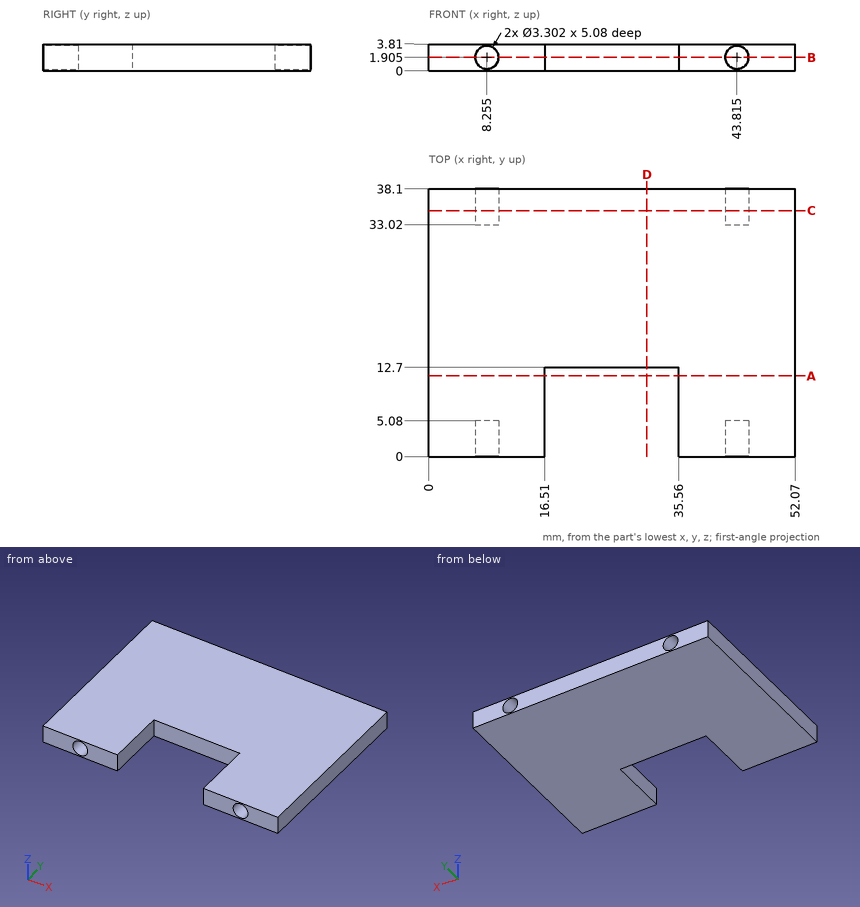
Input: dimensioned drawing with shaded views. Units: mm. Origin: part minimum x, y, z. Coordinates: 2 decimals unless noted, no trailing zeros. Loops run counter-clockwise (first coordinate to the right, second up) from the corner with the lowest first, then second, coordinate; pieces in that order, holes last. Notation, with made-up numbers: M -38,-10.5 L -22,-10.5 A20 cw -22,-6.5 Z; hole C -24,64.25 d2. An arc over 180 degrees is marked long. One line per item, written item: value. Start each with the question number.
1) Cut plane B-B (z = 1.9). Return loops of the section in (x, y), then the cut area to 3 significant figures.
2) Cut plane D-D (x = 31). Return loops of the section in (y, z).
3) Pin query (flat end, axial travel): P1, Ø1.7, axis at x = 44, z = 2.5, coming from the +Y side; P2, Ø2, axis at x = 43.815, z = 1.905, coming from the -Y side; P3, Ø1, axis at x = 19.5, z = 2.5, coming from the -Y side; P4, Ø1.7, axis at x = 44.5, z = 2.5, coming from the -Y side. Return the tip coordinate at first contact, or that it passes through.
4) Cut plane C-C (y = 35). Return loops of the section in (x, z) (3 decimals).
5) Material intervals for L1, parallel to X at y = 2.5, z = 1.95; L2, parallel to X at y = 11, z = 0.35; L3, parallel to Y at x = 31.5, z = 0.9, sorted ascending. Write a range as from..to.
6) Cut plane A-A (y = 11.5). Return loops of the section in (x, z), then the cut area to 3 significant figures.
Evaluation:
1. outline: M 0,0 L 6.6,0 L 6.6,5.08 L 9.91,5.08 L 9.91,0 L 16.51,0 L 16.51,12.7 L 35.56,12.7 L 35.56,0 L 42.16,0 L 42.16,5.08 L 45.47,5.08 L 45.47,0 L 52.07,0 L 52.07,38.1 L 45.47,38.1 L 45.47,33.02 L 42.16,33.02 L 42.16,38.1 L 9.91,38.1 L 9.91,33.02 L 6.6,33.02 L 6.6,38.1 L 0,38.1 Z
1. area: 1,670 mm^2
2. outline: M 12.7,0 L 38.1,0 L 38.1,3.81 L 12.7,3.81 Z
3. P1: y = 33.02
3. P2: y = 5.08
3. P3: y = 12.7
3. P4: y = 0
4. outline: M 0,0 L 52.07,0 L 52.07,3.81 L 0,3.81 Z; hole C 8.255,1.905 d3.302; hole C 43.815,1.905 d3.302
5. L1: 0..6.6, 9.91..16.51, 35.56..42.16, 45.47..52.07
5. L2: 0..16.51, 35.56..52.07
5. L3: 12.7..38.1
6. outline: M 0,0 L 16.51,0 L 16.51,3.81 L 0,3.81 Z; M 35.56,0 L 52.07,0 L 52.07,3.81 L 35.56,3.81 Z
6. area: 126 mm^2
